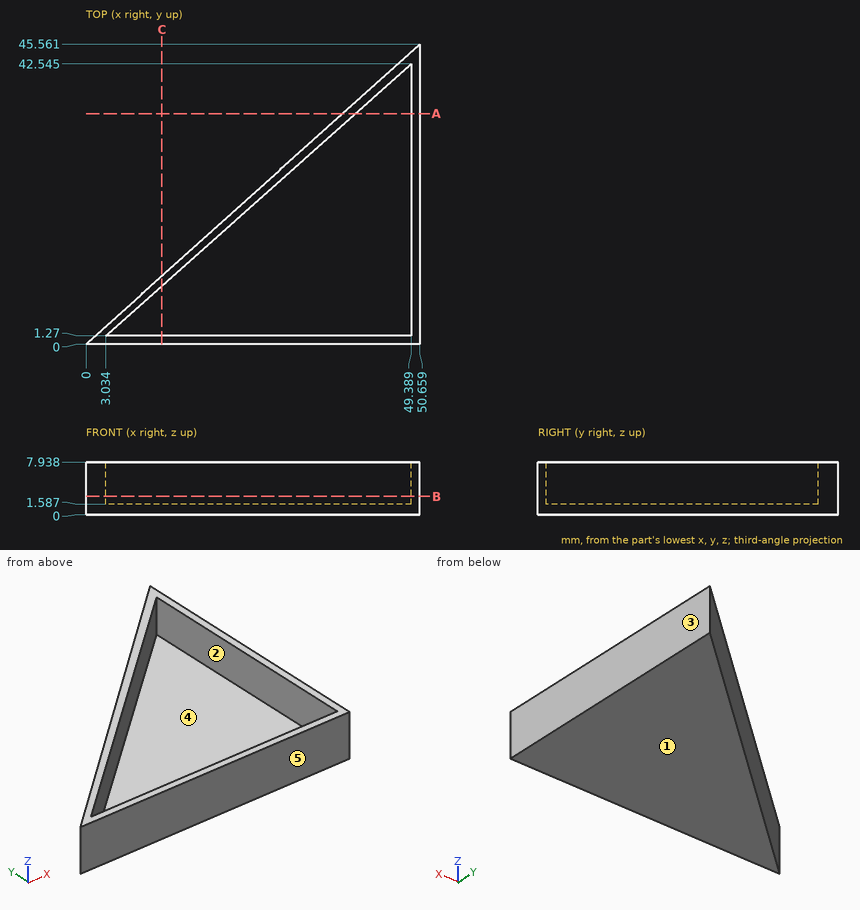
The drawing under review shows one solid part. Ordinate dimensions are in mm from its lowest x, y, z. A direction names the side the tool comes from. Round coordinates to 2 decimals unless told otherwise and drop trailing zeros. Order: outer loops, then holes, each group sorted by start corner. A loop starts at its lowest first (then second) coordinate and runs counter-clockwise, first axis right, second up. Notation, with made-up numbers: (3, 59.5) -> (43, 59.5) arc R14 cw to (43, 84.5) -> close; hole circle Ø3 at (27.25, 10.5). An arc over 180 degrees is marked (long way). Use a Markdown table: item, result.
Item 1: Take a section at C-C (x = 11.5). State the section outline as (y, z) points.
Resolved:
| item | result |
|---|---|
| outline | (0, 0) -> (10.34, 0) -> (10.34, 7.94) -> (8.81, 7.94) -> (8.81, 1.59) -> (1.27, 1.59) -> (1.27, 7.94) -> (0, 7.94) -> close |
Item 2: Take a section at B-B (z = 2.75). State the section outline as (x, y) points (1 decimal).
Resolved:
| item | result |
|---|---|
| outline | (0, 0) -> (50.7, 0) -> (50.7, 45.6) -> close; hole (3, 1.3) -> (49.4, 1.3) -> (49.4, 42.5) -> close |
Item 3: Machinability: for the marked faces 1 and 2, which of the approach directions +Z, -Z, +X, -X, +Y, -Y give a long, thin tool a straight path to every point of the face, cutting with its end or side? Answer none if there is none.
Resolved:
| item | result |
|---|---|
| face 1 | -Z, +X, -X, +Y, -Y |
| face 2 | +Z |
Item 4: Take a section at A-A (y = 35). State the section outline as (x, z) points (1 decimal).
Resolved:
| item | result |
|---|---|
| outline | (38.9, 0) -> (50.7, 0) -> (50.7, 7.9) -> (49.4, 7.9) -> (49.4, 1.6) -> (40.9, 1.6) -> (40.9, 7.9) -> (38.9, 7.9) -> close |
Item 5: Draft analysis for pull direction X (two halves, no side actions). For the marked faces 3, 4 and 5, state which applies: +X half, -X half, draft (parallel to the pull), parting line (faces both ways), or undercut.
Resolved:
| item | result |
|---|---|
| face 3 | +X half |
| face 4 | undercut |
| face 5 | draft |
Item 6: For line 1 along Z through (x, y) = (10.5, 4); line 2 along Y through (x, z) = (33, 5.25); line 3 along X through (y, z) = (16.5, 2) (1 decimal), list the stretches that pass through material, from the lowest coordinate up. Write a range as [from, to].
Resolved:
| item | result |
|---|---|
| line 1 | z = [0, 1.59] |
| line 2 | y = [0, 1.27], [27.95, 29.68] |
| line 3 | x = [18.3, 20.1], [49.4, 50.7] |
Item 7: For pin 1 (2 mm diameter, centred on y = 8, z = 1.5, fed in from -X) (1 decimal); pin 2 (10 mm diameter, centred on x = 14.5, y = 12, fed in from -Z); pin 3 (1.9 mm diameter, centred on x = 31, z = 5, fed in from +Y) (1 decimal); pin 4 (2 mm diameter, centred on x = 14, z = 5, fed in from +Y), all flat-tipped, find the tip position at first contact; note any pin that passes through.
Resolved:
| item | result |
|---|---|
| pin 1 | stops at x = 7.8 |
| pin 2 | stops at z = 0 |
| pin 3 | stops at y = 28.7 |
| pin 4 | stops at y = 13.49 |
